Could you check a few things on this model? Use its own coordinates, in mm. Coordinates: 2 decimals unless noted, no trailing zeros. Loops run counter-clockwise (first coordinate to the right, second up) from the corner with the lowest first, then second, coordinate; pieces in that order, holes last. Notation, with made-up numbers: (-10, 21) - (30, 21) arc R18 ccw to (30, 56) - close; hole circle Ø6 at (1, -14.5). An arc over 180 degrees is marked (long way). One line per item, written item: value. Start each with the question number.
(1) If we section it at C-C on x = 31: Write out the boundary of the cut face in (y, z) (3 decimals), then the cut area to 3 significant figures.
(2) If we section it at A-A on y = 46: Write out the boundary of the cut face in (x, z) (3 decimals), then the cut area to 3 significant figures.
(3) If we mould it in two halves opening along Y, with no side actions, what happens to faces 1 (the face through (22.12, 124.44, 1.61)), 2 (the face through (72.98, 71.4, 1.61)), 3 (the face through (51, 57, 0))? For each: pulls with the +Y half, pulls with the -Y half, needs draft (parallel to the pull), parting line crosses it, or undercut.
(4) If we section it at B-B on z = 2.55: Count the separate pieces of the cut face and the enclosed holes in it, then the cut area to 3 significant figures.
(5) If we section it at D-D on y = 105: Write out the boundary of the cut face in (x, z) (1 decimal), then the cut area to 3 significant figures.
(6) I'm going to push flat-ended pins straight in: P1, Ø7.5, axis at x = 124.41, y = 25.94, coming from the -Z side; P2, Ø1, axis at y = 45.5, z = 1.5, coming from the +X side. Where does each tip first touch, or does it pass through?
(7) If I drill on line 1 along Y through (x, z) = (73, 3); line 2 along Y through (x, z) = (153, 1.65); line 3 along Y through (x, z) = (81, 1.1), over which ranges is the centre line in solid material (lowest first)? Write a range as from..to.
Autodesk Inventor part; units mm, degrees
ref_plane "YZ Plane" through (0, 0, 0) normal (1, 0, 0) x (0, 1, 0)
ref_plane "XZ Plane" through (0, 0, 0) normal (0, 1, 0) x (-1, 0, 0)
ref_plane "XY Plane" through (0, 0, 0) normal (0, 0, 1) x (1, 0, 0)
sketch "Sketch1" plane through (0, 0, 0) normal (0, 0, 1) x (1, 0, 0)
  circle A0 centre (79.9619, 51.3388) radius 7.9375
  line L0 (10.1119, 165.6388) -> (10.1119, 13.2388)
  line L1 (10.1119, 13.2388) -> (162.5119, 13.2388)
  line L2 (162.5119, 13.2388) -> (10.1119, 165.6388)
  point P0 (0, 0)
  dimension "d0" = 15.875
  dimension "d1" = 152.4
  dimension "d2" = 152.4
  dimension "d3" = 38.1
  dimension "d4" = 69.85
extrude "Extrusion1" add sketch "Sketch1" along normal blind 3.175
sketch "Sketch2" plane through (0, 0, 3.175) normal (0, 0, 1) x (1, 0, 0)
  line L0 (10.1119, 13.2388) -> (10.1119, 165.6388)
  line L1 (162.5119, 13.2388) -> (10.1119, 13.2388)
  circle A0 centre (22.8119, 76.7388) radius 3.175
  circle A1 centre (73.6119, 25.9388) radius 3.175
  circle A2 centre (22.8119, 25.9388) radius 3.175
  line L2 (22.8119, 76.7388) -> (22.8119, 25.9388) construction
  line L3 (22.8119, 25.9388) -> (73.6119, 25.9388) construction
  point P0 (0, 0)
  dimension "d7" = 6.35
  dimension "d8" = 12.7
  dimension "d9" = 12.7
  dimension "d10" = 50.8
  dimension "d13" = 50.8
extrude "Extrusion2" cut sketch "Sketch2" against normal through all
sketch "Sketch3" plane through (0, 0, 3.175) normal (0, 0, 1) x (1, 0, 0)
  circle A0 centre (22.8119, 25.9388) radius 3.175
  circle A1 centre (22.8119, 127.5388) radius 3.175
  circle A2 centre (124.4119, 25.9388) radius 3.175
  line L0 (22.8119, 127.5388) -> (22.8119, 25.9388) construction
  line L1 (22.8119, 25.9388) -> (124.4119, 25.9388) construction
  point P0 (0, 0)
  dimension "d14" = 6.35
  dimension "d15" = 101.6
extrude "Extrusion3" cut sketch "Sketch3" against normal through all contours A1 | A2
sketch "Sketch5" plane through (0, 0, 3.175) normal (0, 0, 1) x (1, 0, 0)
  line L0 (10.1119, 165.6388) -> (162.5119, 13.2388)
  arc A0 (33.4951, 142.2556) -> (145.4786, 30.2721) centre (181.5619, 178.3388) ccw
  line L1 (33.4951, 142.2556) -> (145.4786, 30.2721)
  line L2 (10.1119, 13.2388) -> (10.1119, 165.6388)
  point P0 (0, 0)
  dimension "d18" = 152.4
  dimension "d25" = 165.1
  dimension "d26" = 171.45
extrude "Extrusion5" cut sketch "Sketch5" against normal through all
properties part number "CylinderOffsetPlate" material "Aluminum-6061"
Values:
1. outline: (13.239, 0) - (144.751, 0) - (144.751, 3.175) - (13.239, 3.175) - close
1. area: 418 mm2
2. outline: (10.112, 0) - (74.088, 0) - (74.088, 3.175) - (10.112, 3.175) - close; (85.836, 0) - (105.983, 0) - (105.983, 3.175) - (85.836, 3.175) - close
2. area: 267 mm2
3. face 1: undercut
3. face 2: pulls with the +Y half
3. face 3: needs draft
4. separate pieces: 1
4. enclosed holes: 6
4. area: 8,880 mm2
5. outline: (10.1, 0) - (48, 0) - (48, 3.2) - (10.1, 3.2) - close
5. area: 120 mm2
6. P1: stops at z = 0
6. P2: stops at x = 107.76
7. line 1: y = 13.24..22.82, 29.05..47.53, 55.15..71.38
7. line 2: y = 13.24..22.75
7. line 3: y = 13.24..43.47, 59.21..63.83
